```python
from build123d import *

# Parameters (mm, degrees)
F0_W     = 56.6
F0_H     = 91
F1_DEPTH = 15
F2_W     = 51.6
F2_H     = 86
F3_DEPTH = 25
F4_R     = 10
F6_DEPTH = 25


with BuildPart() as f1:
    # F0 (on Top) → F1 (new body)
    with BuildSketch(Plane.XY):
        Rectangle(F0_W, F0_H)
    extrude(amount=F1_DEPTH)

    # F2 (on face) → F3 (cut)
    with BuildSketch(Plane.XY.offset(15)):
        Rectangle(F2_W, F2_H)
    extrude(amount=-F3_DEPTH, mode=Mode.SUBTRACT)

    # F4
    f4_edges = [f1.edges().sort_by_distance(p)[0] for p in [
        (28.3, -45.5, 7.5),
        (28.3, 45.5, 7.5),
        (-28.3, -45.5, 7.5),
        (-28.3, 45.5, 7.5),
        (25.8, 43, 7.5),
        (-25.8, 43, 7.5),
        (-25.8, -43, 7.5),
        (25.8, -43, 7.5),
    ]]
    fillet(f4_edges, radius=F4_R)

    # F5 (on face) → F6 (cut)
    with BuildSketch(Plane.XY.offset(15)):
        Polygon((-28.3, -2), (-28.3, -4), (-25.8, 4), (-25.8, 6), align=None)
    extrude(amount=-F6_DEPTH, mode=Mode.SUBTRACT)


solid = f1.part
```
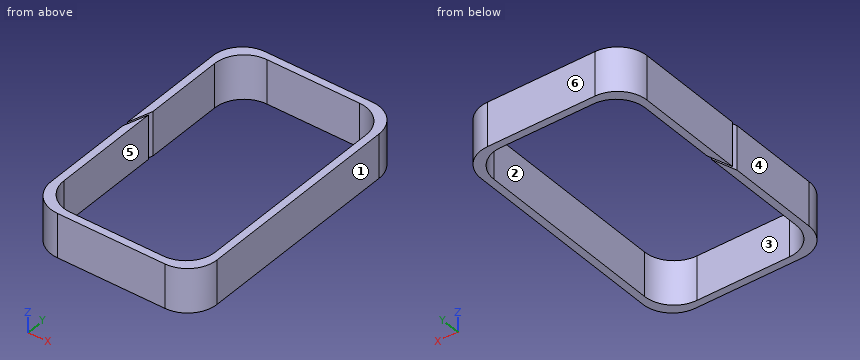
Build history of the part. All positions in model axes, mm. Face numbers are marked on the shaded views. A direction names the side the tool comes from. Coordinates: 2 decimals unless noted, no trailing zeros. Order: outer loops, then holes, each group sorted by start corner. A loop starts at its lowest first (then second) coordinate and runs counter-clockwise, first axis right, second up. Notation, with made-up numbers: M 50,65 L 100,65 A12 ccw 100,87 Z; hole C -27,79 d11. An arc over 180 degrees is marked long. One line per question, with ' | ' between items. Start each with the question number.
1. Wall check: line 1 along X through (y, z) = (-8, 4.5); line 2 along Y through (x, z) = (-6.5, 2.5); line 3 along Y through (x, z) = (18.5, 6.5). Give the ranges that are in metal, low to high. Write a range as [from, to].
2. Tool access for the marked faces 1 and 2: list every direction of +Z, -Z, +X, -X, +Y, -Y with a clear straight run to the whole face (end or side of a thin tool).
3. Cut at C-C (z = 7.5). Write the cut outline in (x, y).
4. Cut at B-B (y = -6). Write the cut outline in (x, z).
5. Cut at A-A (x = -12). Write the cut outline in (y, z), plus the area to 3 significant figures.
6. Mould opens along X. For the marked faces 3, 4, 5 and 6 say: +X half, -X half, draft (parallel to the pull), parting line (faces both ways), or undercut.
The answers:
1) line 1: x = [-28.3, -25.8], [25.8, 28.3] | line 2: y = [-45.5, -43], [43, 45.5] | line 3: y = [-45.5, -42.63], [42.63, 45.5]
2) face 1: +Z, -Z, +X, +Y, -Y | face 2: +Z, -Z
3) outline: M -28.3,-35.5 A10 ccw -18.3,-45.5 L 18.3,-45.5 A10 ccw 28.3,-35.5 L 28.3,35.5 A10 ccw 18.3,45.5 L -18.3,45.5 A10 ccw -28.3,35.5 L -28.3,-2 L -25.8,6 L -25.8,33 A10 cw -15.8,43 L 15.8,43 A10 cw 25.8,33 L 25.8,-33 A10 cw 15.8,-43 L -15.8,-43 A10 cw -25.8,-33 L -25.8,4 L -28.3,-4 Z
4) outline: M -28.3,0 L -25.8,0 L -25.8,15 L -28.3,15 Z; M 25.8,0 L 28.3,0 L 28.3,15 L 25.8,15 Z
5) outline: M -45.5,0 L -43,0 L -43,15 L -45.5,15 Z; M 43,0 L 45.5,0 L 45.5,15 L 43,15 Z | area: 75.0 mm2
6) face 3: undercut | face 4: -X half | face 5: undercut | face 6: draft
